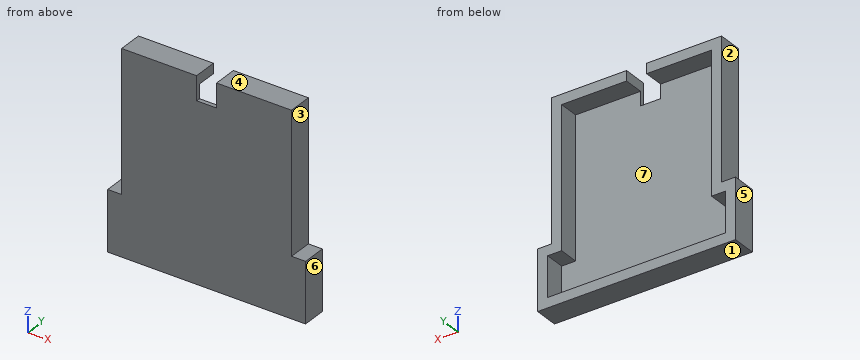
```python
from build123d import *

# Parameters (mm, degrees)
BOSS_EXTRUDE2_DEPTH = 2
BOSS_EXTRUDE3_DEPTH = 12
SKETCH4_W           = 10
SKETCH4_H           = 12
CUT_EXTRUDE1_DEPTH  = 12


with BuildPart() as part:
    # Sketch1 → Boss-Extrude2 (new body)
    with BuildSketch(Plane(origin=(0, 0, 0), x_dir=(1, 0, 0), z_dir=(0, 1, 0))):
        Polygon((30.583615977, 95.111042946), (23.583615977, 95.111042946), (23.583615977, 115.111042946), (112.583615977, 115.111042946), (112.583615977, 95.111042946), (105.583615977, 95.111042946), (105.583615977, 25.111042946), (30.583615977, 25.111042946), align=None)
    extrude(amount=BOSS_EXTRUDE2_DEPTH)

    # Sketch3 → Boss-Extrude3 (add)
    with BuildSketch(Plane(origin=(0, 0, 0), x_dir=(1, 0, 0), z_dir=(0, 1, 0))):
        Polygon((25.583615977, 90.111042946), (25.583615977, 20.111042946), (110.583615977, 20.111042946), (110.583615977, 90.111042946), (117.583615977, 90.111042946), (117.583615977, 120.111042946), (18.583615977, 120.111042946), (18.583615977, 90.111042946), align=None)
        Polygon((30.583615977, 95.111042946), (23.583615977, 95.111042946), (23.583615977, 115.111042946), (112.583615977, 115.111042946), (112.583615977, 95.111042946), (105.583615977, 95.111042946), (105.583615977, 25.111042946), (30.583615977, 25.111042946), align=None, mode=Mode.SUBTRACT)
    extrude(amount=BOSS_EXTRUDE3_DEPTH)

    # Sketch4 → Cut-Extrude1 (cut)
    with BuildSketch(Plane.XY.offset(-20.111042946)):
        with Locations((68.083615977, 6)):
            Rectangle(SKETCH4_W, SKETCH4_H)
    extrude(amount=-CUT_EXTRUDE1_DEPTH, mode=Mode.SUBTRACT)


solid = part.part
```
Verification items for the finished model (mm, model axes). Face numbers are marked on the shaded views. A direction names the side the tool comes from. Give positions to 0.01 mm unless a question says otherwise; leave off trailing zeros. Order: outer loops, then holes, each group sorted by start corner. A loop starts at its lowest first (then second) coordinate and runs counter-clockwise, first axis right, second up. Notation, with made-up numbers: (-9, 40.25) -> (38, 40.25) arc R17 cw to (38, 61.25) -> close; hole circle Ø6 at (-39, 41.5). An arc over 180 degrees is marked (long way). One line per item, written item: value.
(1) Gauge pin test, flat ends, axial feed: pin 1 (1.5 mm diameter, centred on y = 5.5, z = -38.5, fed in from -X); pin 2 (8 mm diameter, centred on x = 72.5, z = -76.5, fed in from +Y); pin 3 (2 mm diameter, centred on y = 1.5, z = -66.5, fed in from +X). Record the tip position at first contact, or that the pin passes through.
Final values:
pin 1: x = 25.58
pin 2: y = 2
pin 3: x = 110.58
(2) Draft check along X on the marked faces 4, 5, 6 and 7. Enter one of: pulls with the +X half, pulls with the -X half, needs draft (parallel to the pull), parting line crosses it, or undercut.
Final values:
face 4: needs draft
face 5: pulls with the -X half
face 6: pulls with the +X half
face 7: undercut
(3) Sectioned sample at A-A on y = 8. Record the cut outline in (x, z).
Final values:
outline: (18.58, -120.11) -> (117.58, -120.11) -> (117.58, -90.11) -> (110.58, -90.11) -> (110.58, -20.11) -> (73.08, -20.11) -> (73.08, -25.11) -> (105.58, -25.11) -> (105.58, -95.11) -> (112.58, -95.11) -> (112.58, -115.11) -> (23.58, -115.11) -> (23.58, -95.11) -> (30.58, -95.11) -> (30.58, -25.11) -> (63.08, -25.11) -> (63.08, -20.11) -> (25.58, -20.11) -> (25.58, -90.11) -> (18.58, -90.11) -> close
(4) Sectioned sample at C-C on x = 46. Record the cut outline in (y, z).
Final values:
outline: (0, -120.11) -> (12, -120.11) -> (12, -115.11) -> (2, -115.11) -> (2, -25.11) -> (12, -25.11) -> (12, -20.11) -> (0, -20.11) -> close
(5) Scan lines: line 1 along X through (y, z) = (9, -114); line 2 along X through (y, z) = (7.5, -56); line 3 along Z through (x, y) = (81, 10.25). Record each from-to range of solid material in increasing order. Write a range as [from, to].
Final values:
line 1: [18.58, 23.58], [112.58, 117.58]
line 2: [25.58, 30.58], [105.58, 110.58]
line 3: [-120.11, -115.11], [-25.11, -20.11]
(6) Sectioned sample at B-B on z = -61. Record the cut outline in (x, y), then the cut area to 3 significant figures.
Final values:
outline: (25.58, 0) -> (110.58, 0) -> (110.58, 12) -> (105.58, 12) -> (105.58, 2) -> (30.58, 2) -> (30.58, 12) -> (25.58, 12) -> close
area: 270 mm^2
(7) Tool access check on the marked faces 1, 2 and 3. Record the directions out of +Z, -Z, +X, -X, +Y, -Y that give a thin tool (end or side, any length) a straight path to the whole face; none if there is none.
Final values:
face 1: -Z, +X, -X, +Y, -Y
face 2: +Z, -X, +Y, -Y
face 3: +Z, +X, +Y, -Y
